```python
from build123d import *

# Parameters (mm, degrees)
SKETCH_1_R      = 1.5
EXTRUDE_1_DEPTH = 2
SKETCH_2_R      = 5
EXTRUDE_2_DEPTH = 10
EXTRUDE_START   = -25
SKETCH_4_R      = 5
EXTRUDE_3_DEPTH = 25
EXTRUDE_4_DEPTH = 7.8
EXTRUDE_START_2 = -7.8
SKETCH_6_R      = 1.6
EXTRUDE_5_DEPTH = 5


with BuildPart() as part:
    # 草图1 → 凸台-拉伸1 (new body)
    with BuildSketch(Plane(origin=(0, 0, 0), x_dir=(1, 0, 0), z_dir=(0, 1, 0))):
        with BuildLine():
            Line((-5, -16), (-5, 16))
            ThreePointArc((-5, 16), (0, 21), (5, 16))
            Line((5, 16), (5, -16))
            ThreePointArc((5, -16), (0, -21), (-5, -16))
        make_face()
        with Locations(Location((0, 16, 0), (0, 0, 270))):
            Circle(SKETCH_1_R, mode=Mode.SUBTRACT)
        Polygon((1.890822132, -12.725), (-1.890822132, -12.725), (-3.781644263, -16), (-1.890822132, -19.275), (1.890822132, -19.275), (3.781644263, -16), align=None, mode=Mode.SUBTRACT)
    extrude(amount=EXTRUDE_1_DEPTH)

    # 草图2 → 凸台-拉伸2 (add)
    with BuildSketch(Plane(origin=(0, 2, 0), x_dir=(1, 0, 0), z_dir=(0, 1, 0))):
        with Locations((0, -16)):
            Circle(SKETCH_2_R)
        Polygon((3.781644263, -16), (1.890822132, -12.725), (-1.890822132, -12.725), (-3.781644263, -16), (-1.890822132, -19.275), (1.890822132, -19.275), align=None, mode=Mode.SUBTRACT)
    extrude(amount=EXTRUDE_2_DEPTH)

    # 草图4 → 凸台-拉伸3 (add)
    with BuildSketch(Plane(origin=(0, 12, 0), x_dir=(1, 0, 0), z_dir=(0, 1, 0)).offset(EXTRUDE_START)):
        with Locations(Location((0, -16, 0), (0, 0, 270))):
            Circle(SKETCH_4_R)
        Polygon((-1.890822132, -12.725), (1.890822132, -12.725), (3.781644263, -16), (1.890822132, -19.275), (-1.890822132, -19.275), (-3.781644263, -16), align=None, mode=Mode.SUBTRACT)
    extrude(amount=EXTRUDE_3_DEPTH)

    # 草图5 → 凸台-拉伸4 (add)
    with BuildSketch(Plane.XZ.offset(13)):
        Polygon((1.890822132, 12.725), (-1.890822132, 12.725), (-3.781644263, 16), (-1.890822132, 19.275), (1.890822132, 19.275), (3.781644263, 16), align=None)
    extrude(amount=-EXTRUDE_4_DEPTH)

    # 草图6 → 凸台-拉伸5 (add)
    with BuildSketch(Plane.XZ.offset(13).offset(EXTRUDE_START_2)):
        with Locations(Location((0, 16, 0), (0, 0, 270))):
            Circle(SKETCH_6_R)
    extrude(amount=-EXTRUDE_5_DEPTH)


solid = part.part
```
Part model, mm, in its own coordinate system. A direction names the side the tool comes from. Coordinates: 2 decimals unless noted, no trailing zeros. Order: outer loops, then holes, each group sorted by start corner. A loop starts at its lowest first (then second) coordinate and runs counter-clockwise, first axis right, second up. Notation, with made-up numbers: (-37.75, 59) - (13.25, 59) arc R13 ccw to (13.25, 84) - close; hole circle Ø7 at (79.25, 26.5). An arc over 180 degrees is marked (long way). Return JSON: item names as keys, results as strings. Group by question number.
Item 1: Cut at D-D (z = -16.5). List the corners of the cut face in (x, y).
Item 2: Pull direction Z, two halves, no side cores. Call faces 4 (the face through (0.07, 0.99, -17.5)), 5 (the face through (0, 0, -3)), 6 (the face through (0, 1, -21)): pulls with the +Z half, pulls with the -Z half, needs draft (parallel to the pull), parting line crosses it, or undercut.
Item 3: Pin check, flat tips, straight feed: pin 1 (1 mm diameter, centred on x = -1, z = 5, fed in from -Y); pin 2 (1 mm diameter, centred on x = 2.5, y = 5, fed in from -Z); pin 3 (3 mm diameter, centred on x = 0.5, y = 4, fed in from -Z). Stop position of each tip, or through.
Item 4: Cut at C-C (y = 5). List the corners of the cut face in (x, z) (3 decimals).
Item 5: Which spindle directions (+Z, -Z, +X, -X, +Y, -Y) get a long thin tool onto all of the face, cutting with end or side? Do faces 1 (the face through (4.41, -0.68, 18.36)), 2 (the face through (0, 3, 19.275)), 3 (the face through (3.3, 12, 14.8)). Say none if no direction does.
Item 6: Cut at A-A (x = 0). List the corners of the cut face in (y, z) (3 decimals), plus the area to 3 significant figures.
Item 7: Cut at B-B (y = 1.25). List the corners of the cut face in (x, z) (3 decimals), plus the area to 3 significant figures.
Item 8: Drill centre lines: probe 1 along X at (y, z) = (0.4, -16); probe 2 along Z at (x, y) = (0.25, 10.75) (3 decimals); probe 3 along Y at (x, z) = (-1.25, -5). Where is each one in solid material? Low to high. Write a range as from..to.
Check values:
{
 "1": {"outline": "(-4.97, 0) - (-1.41, 0) - (-1.41, 2) - (-4.97, 2) - close; (1.41, 0) - (4.97, 0) - (4.97, 2) - (1.41, 2) - close"},
 "2": {"face 4": "undercut", "face 5": "needs draft", "face 6": "pulls with the -Z half"},
 "3": {"pin 1": "stops at y = 0", "pin 2": "stops at z = 11.42", "pin 3": "stops at z = 11"},
 "4": {"outline": "circle Ø10 at (0, 16); hole (-3.782, 16) - (-1.891, 12.725) - (1.891, 12.725) - (3.782, 16) - (1.891, 19.275) - (-1.891, 19.275) - close"},
 "5": {"face 1": "none", "face 2": "+Y", "face 3": "+Z, -Z, +X, -X, +Y"},
 "6": {"outline": "(-13, 11) - (0, 11) - (0, -14.5) - (2, -14.5) - (2, 11) - (12, 11) - (12, 12.725) - (-5.2, 12.725) - (-5.2, 14.4) - (-0.2, 14.4) - (-0.2, 17.6) - (-5.2, 17.6) - (-5.2, 19.275) - (12, 19.275) - (12, 21) - (-13, 21) - close; (0, -21) - (2, -21) - (2, -17.5) - (0, -17.5) - close", "area": "211 mm2"},
 "7": {"outline": "(-5, -16) arc R5 ccw to (5, -16) - (5, 16) arc R5 ccw to (-5, 16) - close; hole (-3.782, 16) - (-1.891, 12.725) - (1.891, 12.725) - (3.782, 16) - (1.891, 19.275) - (-1.891, 19.275) - close; hole circle Ø3 at (0, -16)", "area": "354 mm2"},
 "8": {"probe 1": "x = -5..-1.5, 1.5..5", "probe 2": "z = 11.006..12.725, 19.275..20.994", "probe 3": "y = 0..2"}
}
